```python
from build123d import *

# Parameters (mm, degrees)
SKETCH_W     = 64
SKETCH_H     = 130
PAD_DEPTH    = 13
SKETCH002_W  = 58
SKETCH002_H  = 124
POCKET_DEPTH = 11
SKETCH007_W  = 2.5
SKETCH007_H  = 2.5
PAD001_DEPTH = 3
FILLET_R     = 1.5


with BuildPart() as part:
    # Sketch → Pad (new body)
    with BuildSketch(Plane.XY):
        with Locations((4.5, 22)):
            Rectangle(SKETCH_W, SKETCH_H)
    extrude(amount=PAD_DEPTH)

    # Sketch002 → Pocket (cut)
    with BuildSketch(Plane.XY.offset(13)):
        with Locations((4.5, 22)):
            Rectangle(SKETCH002_W, SKETCH002_H)
    extrude(amount=-POCKET_DEPTH, mode=Mode.SUBTRACT)

    # Sketch007 → Pad001 (new body)
    with BuildSketch(Plane.XY.offset(2)):
        with Locations((-18, 77.5)):
            Rectangle(SKETCH007_W, SKETCH007_H)
        with Locations((27, 77.5)):
            Rectangle(SKETCH007_W, SKETCH007_H)
        with Locations((-18, -17.5)):
            Rectangle(SKETCH007_W, SKETCH007_H)
        with Locations((27, -17.5)):
            Rectangle(SKETCH007_W, SKETCH007_H)
    extrude(amount=PAD001_DEPTH)

    # Fillet
    fillet_edges = [part.edges().sort_by_distance(p)[0] for p in [
        (4.5, 87, 0),
        (-27.5, 22, 0),
        (36.5, 22, 0),
        (4.5, -43, 0),
    ]]
    fillet(fillet_edges, radius=FILLET_R)


solid = part.part
```
Can you work these out from the model? Positions are in its coordinate system, mm. A direction names the side the tool comes from. Coordinates: 2 decimals unless noted, no trailing zeros. Write each loop counter-clockwise with the first axis right and the second up, starting at its lowest first coordinate (ties: lowest second). Pieces come first, ordered by that corner, then holes. Notation, with made-up numbers: M 58,-35 L 101,-35 A30 cw 101,-9 Z; hole C 49,-31 d2. An arc over 180 degrees is marked long. Write item = value, one per line. Start each with the question number.
Q1. If we section it at A-A, the plane z = 8: Write out the boundary of the cut face in (x, y).
Q2. On a 3-axis mill with a long thin cutter (end or side, diameter ignored), from which of +Z, -Z, +X, -X, +Y, -Y can I reach the whole of each face in a straight line? I mean faces 4 (the face through (-27.5, 21, 7)), 5 (the face through (25.75, -18, 3)). Say none if no direction works.
Q3. Thinking about a two-plate mould opening in Y: for faces 1 (the face through (4, -43, 7)), 2 (the face through (-16.75, -18, 3)), 3 (the face through (4, 23, 0)), which applies, released by +Y, released by -Y, zero draft, split by the parting line, or undercut?
Q4. If I drill on L1, parallel to Y at x = -22.5, z = 6; L2, parallel to X at y = -22.5, z = 3.75; L3, parallel to Z at x = 23.5, y = 80, over which ranges is the centre line in solid material (lowest first)? Write a range as [from, to].
Q5. If we section it at C-C, the plane y = -32: Write out the boundary of the cut face in (x, z), then the cut area to 3 significant figures.
Q6. If we section it at B-B, the plane x = -1: Write out the boundary of the cut face in (y, z), then the cut area to 3 significant figures.
Q7. I'm going to push a flat-ended pin straight in: pin 1 (1.2 mm diameter, centred on x = 27.5, y = -18, fed in from +Z). Where does the tip first touch, or does it pass through?
Check sheet entries:
q1.outline = M -27.5,-43 L 36.5,-43 L 36.5,87 L -27.5,87 Z; hole M -24.5,-40 L 33.5,-40 L 33.5,84 L -24.5,84 Z
q2.face_4 = +Z, -Z, -X, +Y, -Y
q2.face_5 = +Z
q3.face_1 = released by -Y
q3.face_2 = undercut
q3.face_3 = zero draft
q4.L1 = [-43, -40], [84, 87]
q4.L2 = [-27.5, -24.5], [33.5, 36.5]
q4.L3 = [0, 2]
q5.outline = M -27.5,1.5 A1.5 ccw -26,0 L 35,0 A1.5 ccw 36.5,1.5 L 36.5,13 L 33.5,13 L 33.5,2 L -24.5,2 L -24.5,13 L -27.5,13 Z
q5.area = 193 mm²
q6.outline = M -43,1.5 A1.5 ccw -41.5,0 L 85.5,0 A1.5 ccw 87,1.5 L 87,13 L 84,13 L 84,2 L -40,2 L -40,13 L -43,13 Z
q6.area = 325 mm²
q7.pin_1 = 5
